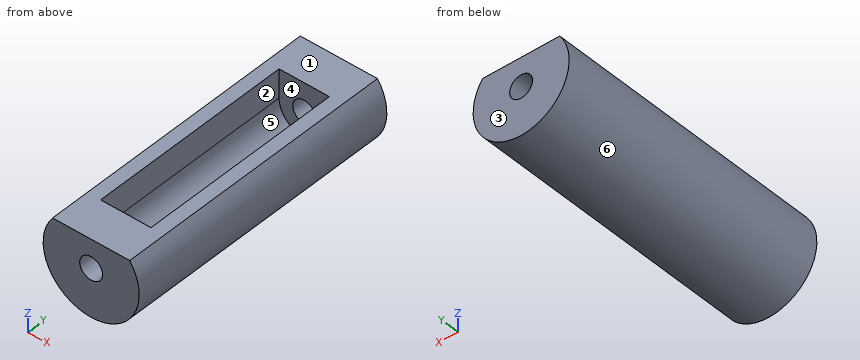
```python
from build123d import *

# Parameters (mm, degrees)
SKETCH1_R           = 2
BOSS_EXTRUDE1_DEPTH = 7
BOSS_EXTRUDE3_DEPTH = 36
SKETCH5_R           = 2
BOSS_EXTRUDE4_DEPTH = 7


with BuildPart() as part:
    # Sketch1 → Boss-Extrude1 (new body)
    with BuildSketch(Plane(origin=(0, 0, 0), x_dir=(1, 0, 0), z_dir=(0, 1, 0))):
        with BuildLine():
            Line((6.749814812, -5), (-6.749814812, -5))
            ThreePointArc((-6.749814812, -5), (0, 8.4), (6.749814812, -5))
        make_face()
        with Locations(Location((0, 0, 0), (0, 0, 270))):
            Circle(SKETCH1_R, mode=Mode.SUBTRACT)
    extrude(amount=BOSS_EXTRUDE1_DEPTH)

    # Sketch3 → Boss-Extrude3 (add)
    with BuildSketch(Plane(origin=(0, 7, 0), x_dir=(1, 0, 0), z_dir=(0, 1, 0))):
        with BuildLine():
            Line((-4.4, 0), (-4.4, -5))
            Line((-4.4, -5), (-6.749814812, -5))
            ThreePointArc((-6.749814812, -5), (0, 8.4), (6.749814812, -5))
            Line((6.749814812, -5), (4.4, -5))
            Line((4.4, -5), (4.4, 0))
            ThreePointArc((4.4, 0), (0, 4.4), (-4.4, 0))
        make_face()
    extrude(amount=BOSS_EXTRUDE3_DEPTH)

    # Sketch5 → Boss-Extrude4 (add)
    with BuildSketch(Plane(origin=(0, 43, 0), x_dir=(1, 0, 0), z_dir=(0, 1, 0))):
        with BuildLine():
            Line((6.749814812, -5), (-6.749814812, -5))
            ThreePointArc((-6.749814812, -5), (0, 8.4), (6.749814812, -5))
        make_face()
        with Locations(Location((0, 0, 0), (0, 0, 270))):
            Circle(SKETCH5_R, mode=Mode.SUBTRACT)
    extrude(amount=BOSS_EXTRUDE4_DEPTH)


solid = part.part
```
Can you work these out from the model? Positions are in its coordinate system, mm. Face numbers are marked on the shaded views. A direction names the side the tool comes from. Round coordinates to 2 decimals unless told otherwise and drop trailing zeros. Loops run counter-clockwise (first coordinate to the right, second up) from the corner with the lowest first, then second, coordinate; pieces in that order, holes last. Notation, with made-up numbers: (-31.5, 35.25) -> (0.5, 35.25) arc R23 cw to (0.5, 66.25) -> close; hole circle Ø9 at (-16.5, 67). An arc over 180 degrees is marked (long way). One line per item, written item: value. Start each with the question number.
1. If we mould it in two halves opening along X, with no side actions, what happens to the marked faces 3, 4, 5 and 6? For each: pulls with the +X half, pulls with the -X half, needs draft (parallel to the pull), parting line crosses it, or undercut.
2. If we section it at C-C, the plane y = 17.5: Write out the boundary of the cut face in (x, z), then the cut area to 3 significant figures.
3. For pin 1 (2 mm diameter, centred on y = 23, z = -5, fed in from +X); pin 2 (2.5 mm diameter, centred on y = 19, z = 2, fed in from +X); pin 3 (2 mm diameter, centred on x = 4.5, z = 2.5, fed in from -Y); pin 4 (4 mm diameter, centred on y = 33, z = 3.5, fed in from -X) (3 decimals), each with a flat end and sliding along its axis, tell me the tip position at first contact or that it passes through.
4. For the marked faces 1 and 2, which set-ups out of +Z, -Z, +X, -X, +Y, -Y let a thin tool reach every point of the face, with its end or its side?
5. If we section it at D-D, the plane x = 2.5: Write out the boundary of the cut face in (y, z).
6. If I drill on probe 1 along Y at (x, z) = (-2.5, -0.5); probe 2 along X at (y, z) = (2, 0); probe 3 along X at (y, z) = (33.5, 3.5), over which ranges is the centre line in solid material (lowest first)?
7. If we section it at A-A, the plane x = 0: Write out the boundary of the cut face in (y, z), then the cut area to 3 significant figures.
8. If we section it at B-B, the plane z = 3.5: Write out the boundary of the cut face in (x, y), then the cut area to 3 significant figures.
Calculated:
1. face 3: needs draft
1. face 4: undercut
1. face 5: undercut
1. face 6: parting line crosses it
2. outline: (-6.75, 5) arc R8.4 ccw (long way) to (6.75, 5) -> (4.4, 5) -> (4.4, 0) arc R4.4 cw to (-4.4, 0) -> (-4.4, 5) -> close
2. area: 115 mm²
3. pin 1: stops at x = 7.39
3. pin 2: stops at x = 8.37
3. pin 3: stops at y = 0
3. pin 4: stops at x = -8.265
4. face 1: +Z, +X, -X, +Y, -Y
4. face 2: +Z
5. outline: (0, -8.02) -> (50, -8.02) -> (50, 5) -> (43, 5) -> (43, -3.62) -> (7, -3.62) -> (7, 5) -> (0, 5) -> close
6. probe 1: y = 0 to 7, 43 to 50
6. probe 2: x = -8.4 to -2, 2 to 8.4
6. probe 3: x = -7.64 to -4.4, 4.4 to 7.64
7. outline: (0, -8.4) -> (50, -8.4) -> (50, -2) -> (43, -2) -> (43, -4.4) -> (7, -4.4) -> (7, -2) -> (0, -2) -> close; (0, 2) -> (7, 2) -> (7, 5) -> (0, 5) -> close; (43, 2) -> (50, 2) -> (50, 5) -> (43, 5) -> close
7. area: 276 mm²
8. outline: (-7.64, 0) -> (7.64, 0) -> (7.64, 50) -> (-7.64, 50) -> close; hole (-4.4, 7) -> (4.4, 7) -> (4.4, 43) -> (-4.4, 43) -> close
8. area: 447 mm²
